from build123d import *

# Parameters (mm, degrees)
SKETCH_2_R          = 1.5
CUT_EXTRUDE_1_DEPTH = 10


with BuildPart() as part:
    # 草图1 → 旋转1 (revolve)
    with BuildSketch(Plane.XY, mode=Mode.PRIVATE) as revolve_1_sk:
        Polygon((0, 98), (2.5, 98), (2.5, 82), (8.75, 82), (8.75, 77), (21, 77), (21, 70.5), (22, 70.5), (22, 36.5), (21, 36.5), (21, 10.5), (7.5, 10.5), (7.5, 5), (5, 5), (5, 0), (0, 0), align=None)
    revolve(revolve_1_sk.sketch.rotate(Axis((0, 120.576266676, 0), (0, -1, 0)), 90), axis=Axis((0, 120.576266676, 0), (0, -1, 0)))

    # 草图2 → 切除-拉伸1 (cut)
    with BuildSketch(Plane(origin=(0, 77, 0), x_dir=(1, 0, 0), z_dir=(0, 1, 0))):
        with Locations(Location((14.5, 0, 0), (0, 0, 270))):
            Circle(SKETCH_2_R)
        with Locations(Location((-14.5, 0, 0), (0, 0, 90))):
            Circle(SKETCH_2_R)
    extrude(amount=-CUT_EXTRUDE_1_DEPTH, mode=Mode.SUBTRACT)


solid = part.part
The model under review builds one solid part; all positions refer to its coordinate system, in mm. A direction names the side the tool comes from. Round coordinates to 2 decimals unless told otherwise and drop trailing zeros. Order: outer loops, then holes, each group sorted by start corner. A loop starts at its lowest first (then second) coordinate and runs counter-clockwise, first axis right, second up. Notation, with made-up numbers: (-23, 77) -> (21, 77) arc R10 ccw to (21, 88) -> close; hole circle Ø9 at (89.25, -8). An arc over 180 degrees is marked (long way). Write item = value, one per line. Start each with the question number.
Item 1: Mouldability with a two-part tool opening along X and no side actions: class faces 1 (the face through (0, 77, -9)), 2 (the face through (-14.95, 72.07, -1.43)), 3 (the face through (-6.31, 73.7, 20.03)) as released by +X, released by -X, zero draft, split by the parting line, or undercut.
Item 2: Clearance check with flat-ended pins moving along their axes: pin 1 Ø0.9 at (x, z) = (15, 0.5) entering from +Y; pin 2 Ø4 at (y, z) = (57.5, 13) entering from -X; pin 3 Ø10 at (y, z) = (38, -5.5) entering from -X. State where each tip first meets the part, or that it passes through.
Item 3: For faces 4 (the face through (0, 0, 0)), 5 (the face through (0, 2, -5)), 6 (the face through (15, 67, 0)), list the 3-axis set-ups (+Z, -Z, +X, -X, +Y, -Y) from which the entire face can be reached by the end or side of a thin tool; tool diameter is ignored.
Item 4: Consider section B-B on z = 14.5. Write out the cut boundary in (x, y).
Item 5: Consider section A-A on x = 0. Write out the cut boundary in (y, z), plus the area to 3 significant figures.
Item 6: Consider section D-D on x = 17.5. Write out the cut boundary in (y, z), plus the area to 3 significant figures.
Item 7: Consider section C-C on y = 30. Write out the cut boundary in (x, z), plus the area to 3 significant figures.
Item 8: For line 1 along X through (y, z) = (73, 0); line 2 along X through (y, z) = (70.25, 0); line 3 along Y through (x, z) = (17.5, 8.5), list the stretches that pass through material, from the lowest coordinate up.
Conclusion:
q1.face_1 = zero draft
q1.face_2 = undercut
q1.face_3 = split by the parting line
q2.pin_1 = 67
q2.pin_2 = -19.05
q2.pin_3 = -21.99
q3.face_4 = +Z, -Z, +X, -X, -Y
q3.face_5 = -Y
q3.face_6 = +Y
q4.outline = (-16.55, 36.5) -> (-15.19, 36.5) -> (-15.19, 10.5) -> (15.19, 10.5) -> (15.19, 36.5) -> (16.55, 36.5) -> (16.55, 70.5) -> (15.19, 70.5) -> (15.19, 77) -> (-15.19, 77) -> (-15.19, 70.5) -> (-16.55, 70.5) -> close
q5.outline = (0, -5) -> (5, -5) -> (5, -7.5) -> (10.5, -7.5) -> (10.5, -21) -> (36.5, -21) -> (36.5, -22) -> (70.5, -22) -> (70.5, -21) -> (77, -21) -> (77, -8.75) -> (82, -8.75) -> (82, -2.5) -> (98, -2.5) -> (98, 2.5) -> (82, 2.5) -> (82, 8.75) -> (77, 8.75) -> (77, 21) -> (70.5, 21) -> (70.5, 22) -> (36.5, 22) -> (36.5, 21) -> (10.5, 21) -> (10.5, 7.5) -> (5, 7.5) -> (5, 5) -> (0, 5) -> close
q5.area = 3,160 mm2
q6.outline = (10.5, -11.61) -> (36.5, -11.61) -> (36.5, -13.33) -> (70.5, -13.33) -> (70.5, -11.61) -> (77, -11.61) -> (77, 11.61) -> (70.5, 11.61) -> (70.5, 13.33) -> (36.5, 13.33) -> (36.5, 11.61) -> (10.5, 11.61) -> close
q6.area = 1,660 mm2
q7.outline = circle Ø42 at (0, 0)
q7.area = 1,390 mm2
q8.line_1 = -21 to -16, -13 to 13, 16 to 21
q8.line_2 = -22 to -16, -13 to 13, 16 to 22
q8.line_3 = 10.5 to 77
